from build123d import *

# Parameters (mm, degrees)
CROQUIS1_R              = 3
SALIENTE_EXTRUIR1_DEPTH = 5
CROQUIS2_R              = 5.000500025
SALIENTE_EXTRUIR2_DEPTH = 10
CROQUIS3_R              = 5.000500025
CROQUIS3_R_2            = 3
SALIENTE_EXTRUIR3_DEPTH = 4.8
SALIENTE_EXTRUIR4_DEPTH = 14


with BuildPart() as part:
    # Croquis1 → Saliente-Extruir1 (new body)
    with BuildSketch(Plane.XY):
        Circle(CROQUIS1_R)
        with BuildLine():
            Line((-1.29614814, 1.1), (1.29614814, 1.1))
            ThreePointArc((1.29614814, 1.1), (0, -1.7), (-1.29614814, 1.1))
        make_face(mode=Mode.SUBTRACT)
    extrude(amount=SALIENTE_EXTRUIR1_DEPTH)

    # Croquis2 → Saliente-Extruir2 (add)
    with BuildSketch(Plane(origin=(0, 0, 0), x_dir=(-1, 0, 0), z_dir=(0, 0, -1))):
        Circle(CROQUIS2_R)
    extrude(amount=SALIENTE_EXTRUIR2_DEPTH)

    # Croquis3 → Saliente-Extruir3 (add)
    with BuildSketch(Plane.XY):
        Circle(CROQUIS3_R)
        Circle(CROQUIS3_R_2, mode=Mode.SUBTRACT)
    extrude(amount=SALIENTE_EXTRUIR3_DEPTH)

    # Croquis4 → Saliente-Extruir4 (add)
    with BuildSketch(Plane(origin=(0, 0, -10), x_dir=(-1, 0, 0), z_dir=(0, 0, -1))):
        Polygon((-1.5, 4.442041839), (1.5, 4.442041839), (3, 17.942041839), (-3, 17.942041839), align=None)
        Polygon((17.038264028, 6.372944708), (14.038264028, 11.569097131), (3.096921077, 3.520059025), (4.596921077, 0.921982814), align=None)
        Polygon((14.038264028, -11.569097131), (17.038264028, -6.372944708), (4.596921077, -0.921982814), (3.096921077, -3.520059025), align=None)
        Polygon((-3, -17.942041839), (3, -17.942041839), (1.5, -4.442041839), (-1.5, -4.442041839), align=None)
        Polygon((-17.038264028, -6.372944708), (-14.038264028, -11.569097131), (-3.096921077, -3.520059025), (-4.596921077, -0.921982814), align=None)
        Polygon((-14.038264028, 11.569097131), (-17.038264028, 6.372944708), (-4.596921077, 0.921982814), (-3.096921077, 3.520059025), align=None)
    extrude(amount=-SALIENTE_EXTRUIR4_DEPTH)

    # Croquis6 → Revolución2 (revolve)
    with BuildSketch(Plane(origin=(0, 0, 0), x_dir=(0, 0, -1), z_dir=(1, 0, 0)), mode=Mode.PRIVATE) as revoluci_n2_sk:
        with BuildLine():
            Line((10, 17.942041839), (10, 18.942041839))
            ThreePointArc((10, 18.942041839), (3.5, 19.473700095), (-3, 18.942041839))
            Line((-3, 18.942041839), (-3, 17.942041839))
            Line((-3, 17.942041839), (10, 17.942041839))
        make_face()
    revolve(revoluci_n2_sk.sketch.rotate(Axis((0, 0, 4), (0, 0, -1)), 90), axis=Axis((0, 0, 4), (0, 0, -1)))


solid = part.part
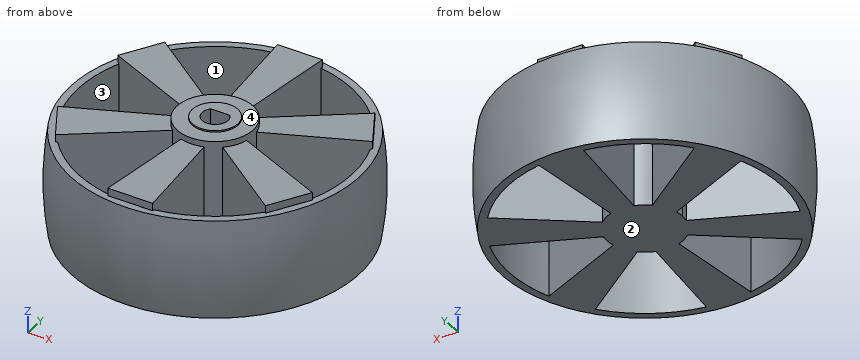
The listing builds one solid part. Answer for the finished solid, in the listing's coordinates (mm). Face numbers are marked on the shaded views. A direction names the side the tool comes from. Coordinates: 2 decimals unless noted, no trailing zeros. Write each loop counter-clockwise with the first axis right and the second up, starting at its lowest first coordinate (ties: lowest second). Pieces come first, ordered by that corner, then holes. Notation, with made-up numbers: (17, -31) - (26, -31) arc R7 cw to (26, -27) - close; hole circle Ø7 at (11.5, -18.5). An arc over 180 degrees is marked (long way). Return JSON: item names as keys, results as strings.
1. Which of the six approach directions +Z, -Z, +X, -X, +Y, -Y give full straight-line access (tool end or side, diameter ignored) to the marked faces 3 and 4?
Final values:
{"face 3": "+Z, -Z", "face 4": "+Z"}
2. For a pull along X with two mould halves and no side action, classify the marked faces 1 and 2 as +X half, -X half, draft (parallel to the pull), parting line (faces both ways), or undercut.
Final values:
{"face 1": "undercut", "face 2": "draft"}
3. Each of these flat-tipped pins is pushed along its axis until it touches: pin 1 Ø1.5 at (y, z) = (-14.5, 1) entering from +X; pin 2 Ø8 at (x, z) = (-6.5, -2.5) entering from +Y; pin 3 Ø1.1 at (x, z) = (0, 3.5) entering from +Y. Where does it stop, or does it pass through?
Final values:
{"pin 1": "x = 13.44", "pin 2": "y = 19.31", "pin 3": "y = 18.95"}
4. The part is cut by section A-A on z = 3.5. Determine the outline of the cut face in (x, y).
Final values:
{"outline": "(-17.04, -6.37) - (-14.04, -11.57) - (-3.35, -3.71) arc R5 ccw to (-1.54, -4.76) - (-3, -17.94) - (3, -17.94) - (1.54, -4.76) arc R5 ccw to (3.35, -3.71) - (14.04, -11.57) - (17.04, -6.37) - (4.89, -1.05) arc R5 ccw to (4.89, 1.05) - (17.04, 6.37) - (14.04, 11.57) - (3.35, 3.71) arc R5 ccw to (1.54, 4.76) - (3, 17.94) - (-3, 17.94) - (-1.54, 4.76) arc R5 ccw to (-3.35, 3.71) - (-14.04, 11.57) - (-17.04, 6.37) - (-4.89, 1.05) arc R5 ccw to (-4.89, -1.05) - close; hole (-1.3, 1.1) arc R1.7 ccw (long way) to (1.3, 1.1) - close"}
5. The part is cut by section B-B on x = 4. Count the separate pieces of the cut face and the enclosed holes in it, then the cut area to 3 significant figures.
Final values:
{"separate pieces": "3", "enclosed holes": "0", "area": "158 mm^2"}
6. Consider line 1 along X through (y, z) = (0, 4); line 2 along X through (y, z) = (7, -9.5); line 3 along Y through (x, z) = (-12, 0.25). Determine where each line is inside the solid, lowest interval first.
Final values:
{"line 1": "-5 to -1.7, 1.7 to 5", "line 2": "-17.69 to -7.83, -1.78 to 1.78, 7.83 to 17.69", "line 3": "-15.11 to -13.34, -10.07 to -4.17, 4.17 to 10.07, 13.34 to 15.11"}
